```python
from build123d import *


with BuildPart() as part:
    # Esquisse1 → Révolution1 (revolve)
    with BuildSketch(Plane.XY, mode=Mode.PRIVATE) as r_volution1_sk:
        with BuildLine():
            Line((-3.5, 3), (-3.3, 3))
            Line((-3.3, 3), (-3.3, 4.5))
            Line((-3.3, 4.5), (-3.5, 4.5))
            Line((-3.5, 4.5), (-3.5, 6.5))
            Line((-3.5, 6.5), (-2.5, 6.5))
            ThreePointArc((-2.5, 6.5), (0, 4.75), (2.5, 6.5))
            Line((2.5, 6.5), (3.5, 6.5))
            Line((3.5, 6.5), (3.5, 4.5))
            Line((3.5, 4.5), (3.3, 4.5))
            Line((3.3, 4.5), (3.3, 3))
            Line((3.3, 3), (3.5, 3))
            Line((3.5, 3), (3.5, 2))
            Line((3.5, 2), (-3.5, 2))
            Line((-3.5, 2), (-3.5, 3))
        make_face()
    revolve(r_volution1_sk.sketch.rotate(Axis((-3.5, 0, 0), (1, 0, 0)), 90), axis=Axis((-3.5, 0, 0), (1, 0, 0)))


solid = part.part
```
Check sheet for the modelled part. Datum: model origin and axes. Units: mm. A direction names the side the tool comes from. Give positions to 0.01 mm unless a question says otherwise; leave off trailing zeros. Loops run counter-clockwise (first coordinate to the right, second up) from the corner with the lowest first, then second, coordinate; pieces in that order, holes last. Notation, with made-up numbers: M 1.25,76.25 L 30.25,76.25 A23 cw 30.25,97.25 Z; hole C -20,60 d3. An arc over 180 degrees is marked long. Answer in a Markdown table with one row per item.
1) Cross-section at A-A (z = 0). Enter the section's corners in (x, y), plus the area to 3 significant figures.
Solutions:
| item | result |
|---|---|
| outline | M -3.5,-6.5 L -2.5,-6.5 A2.66 cw 2.5,-6.5 L 3.5,-6.5 L 3.5,-4.5 L 3.3,-4.5 L 3.3,-3 L 3.5,-3 L 3.5,-2 L -3.5,-2 L -3.5,-3 L -3.3,-3 L -3.3,-4.5 L -3.5,-4.5 Z; M -3.5,2 L 3.5,2 L 3.5,3 L 3.3,3 L 3.3,4.5 L 3.5,4.5 L 3.5,6.5 L 2.5,6.5 A2.66 cw -2.5,6.5 L -3.5,6.5 L -3.5,4.5 L -3.3,4.5 L -3.3,3 L -3.5,3 Z |
| area | 49.1 mm^2 |
2) Depth check by flat-ended pin: pin 1 (3.5 mm diameter, centred on y = 0, z = 0, fed in from +X); pin 2 (4 mm diameter, centred on x = -1, z = 4.5, fed in from +Y); pin 3 (2 mm diameter, centred on x = 1, z = 5, fed in from +Y). Enter the tip coordinate at first touch or a pass-through.
Solutions:
| item | result |
|---|---|
| pin 1 | passes through |
| pin 2 | stops at y = 5.67 |
| pin 3 | stops at y = 3.23 |
3) Thickness scan on line 1 (Y direction, x = 3.4, z = 0); line 2 (X direction, y = 2, z = -2.75); line 3 (Y direction, x = 1.5, z = 0.75). Record the ranges inside material, lowest first.
Solutions:
| item | result |
|---|---|
| line 1 | y = -6.5 to -4.5, -3 to -2, 2 to 3, 4.5 to 6.5 |
| line 2 | x = -3.3 to 3.3 |
| line 3 | y = -5.16 to -1.85, 1.85 to 5.16 |
4) Mould release check, pull along Y, two halves, no side actions. Record for faces 1 (the face through (-2.993, 3.955, -5.158)), 2 (the face through (0, 2, 0)), 3 (the face through (3.5, -4.42, -1.54)): released by +Y, released by -Y, zero draft, split by the parting line, or undercut.
Solutions:
| item | result |
|---|---|
| face 1 | split by the parting line |
| face 2 | undercut |
| face 3 | zero draft |
5) Cross-section at C-C (x = 0). Enter the section's corners in (y, z).
Solutions:
| item | result |
|---|---|
| outline | C 0,0 d9.5; hole C 0,0 d4 |
6) Tool access check on faces 4 (the face through (3.5, 2, 1)), 5 (the face through (-3.3, 3, -1)), 6 (the face through (3.3, 3, 1)). Record the directions out of +Z, -Z, +X, -X, +Y, -Y that give a thin tool (end or side, any length) a straight path to the whole face; none if there is none.
Solutions:
| item | result |
|---|---|
| face 4 | +Z, -Z, +X, +Y, -Y |
| face 5 | -X |
| face 6 | +X |
